from build123d import *

# Parameters (mm, degrees)
SKETCH1_W                = 250
SKETCH1_H                = 115
SKETCH1_R                = 8.5
SKETCH1_W_2              = 83
SKETCH1_H_2              = 55
BOSS_EXTRUDE1_DEPTH      = 10
SKETCH2_W                = 230
SKETCH2_H                = 95
SKETCH2_W_2              = 214
SKETCH2_H_2              = 79
BOSS_EXTRUDE2_DEPTH      = 15
SKETCH3_W                = 25
SKETCH3_H                = 25
CUT_EXTRUDE1_DEPTH       = 7
SKETCH4_W                = 93
SKETCH4_H                = 65
SKETCH4_W_2              = 83
SKETCH4_H_2              = 55
CUT_EXTRUDE2_DEPTH       = 5
SKETCH5_W                = 7
SKETCH5_H                = 5
SKETCH5_W_2              = 10
BOSS_EXTRUDE3_DEPTH      = 8
SKETCH7_W                = 7
SKETCH7_H                = 30
SKETCH7_W_2              = 10
BOSS_EXTRUDE4_DEPTH      = 5
SKETCH8_W                = 5.6
SKETCH8_H                = 2.8
CUT_EXTRUDE7_DEPTH       = 6.6
SKETCH9_W                = 5.6
SKETCH9_H                = 2.8
CUT_EXTRUDE8_DEPTH       = 6.6
CUT_EXTRUDE9_DEPTH       = 139.38457284
CUT_EXTRUDE9_DEPTH_BACK  = 139.38457284
SKETCH10_R               = 1.65
SKETCH11_R               = 1.65
BOSS_EXTRUDE5_DEPTH      = 3
SKETCH12_W               = 10
SKETCH12_H               = 0.5
CUT_EXTRUDE10_DEPTH      = 3
SKETCH13_W               = 30
SKETCH13_H               = 8
CUT_EXTRUDE11_DEPTH      = 6
SKETCH14_W               = 5.6
SKETCH14_H               = 2.8
CUT_EXTRUDE12_DEPTH      = 6.6
CUT_EXTRUDE13_DEPTH      = 139.222610307
CUT_EXTRUDE13_DEPTH_BACK = 139.222610307
SKETCH15_R               = 1.65
SKETCH16_W               = 5.6
SKETCH16_H               = 2.8
CUT_EXTRUDE14_DEPTH      = 6.6
CUT_EXTRUDE15_DEPTH      = 139.222610307
CUT_EXTRUDE15_DEPTH_BACK = 139.222610307
SKETCH17_R               = 1.65
SKETCH18_R               = 1.65
BOSS_EXTRUDE6_DEPTH      = 4
CHAMFER1_SIZE            = 15
CHAMFER2_SIZE            = 5
FILLET1_R                = 5


with BuildPart() as part:
    # Sketch1 → Boss-Extrude1 (new body)
    with BuildSketch(Plane(origin=(0, 0, 0), x_dir=(1, 0, 0), z_dir=(0, 1, 0))):
        Rectangle(SKETCH1_W, SKETCH1_H)
        with Locations(Location((23, 15, 0), (0, 0, 270))):
            Circle(SKETCH1_R, mode=Mode.SUBTRACT)
        with Locations(Location((58, 15, 0), (0, 0, 270))):
            Circle(SKETCH1_R, mode=Mode.SUBTRACT)
        with Locations(Location((23, -15, 0), (0, 0, 270))):
            Circle(SKETCH1_R, mode=Mode.SUBTRACT)
        with Locations(Location((58, -15, 0), (0, 0, 270))):
            Circle(SKETCH1_R, mode=Mode.SUBTRACT)
        with Locations(Location((93, 0, 0), (0, 0, 270))):
            Circle(SKETCH1_R, mode=Mode.SUBTRACT)
        with Locations((-53.5, 0)):
            Rectangle(SKETCH1_W_2, SKETCH1_H_2, mode=Mode.SUBTRACT)
    extrude(amount=BOSS_EXTRUDE1_DEPTH)

    # Sketch2 → Boss-Extrude2 (add)
    with BuildSketch(Plane.XZ):
        Rectangle(SKETCH2_W, SKETCH2_H)
        Rectangle(SKETCH2_W_2, SKETCH2_H_2, mode=Mode.SUBTRACT)
    extrude(amount=BOSS_EXTRUDE2_DEPTH)

    # Sketch3 → Cut-Extrude1 (cut)
    with BuildSketch(Plane.XZ):
        with Locations((23, 15)):
            Rectangle(SKETCH3_W, SKETCH3_H)
        with Locations((58, 15)):
            Rectangle(SKETCH3_W, SKETCH3_H)
        with Locations((23, -15)):
            Rectangle(SKETCH3_W, SKETCH3_H)
        with Locations((58, -15)):
            Rectangle(SKETCH3_W, SKETCH3_H)
        with Locations((93, 0)):
            Rectangle(SKETCH3_W, SKETCH3_H)
    extrude(amount=-CUT_EXTRUDE1_DEPTH, mode=Mode.SUBTRACT)

    # Sketch4 → Cut-Extrude2 (cut)
    with BuildSketch(Plane.XZ):
        with Locations((-53.5, 0)):
            Rectangle(SKETCH4_W, SKETCH4_H)
        with Locations((-53.5, 0)):
            Rectangle(SKETCH4_W_2, SKETCH4_H_2, mode=Mode.SUBTRACT)
    extrude(amount=-CUT_EXTRUDE2_DEPTH, mode=Mode.SUBTRACT)

    # Sketch5 → Boss-Extrude3 (add)
    with BuildSketch(Plane.XZ):
        with Locations((-103.5, 17.5)):
            Rectangle(SKETCH5_W, SKETCH5_H)
        with Locations((-103.5, -17.5)):
            Rectangle(SKETCH5_W, SKETCH5_H)
        with Locations((-2, 17.853765276)):
            Rectangle(SKETCH5_W_2, SKETCH5_H)
        with Locations((-2, -17.146234724)):
            Rectangle(SKETCH5_W_2, SKETCH5_H)
    extrude(amount=BOSS_EXTRUDE3_DEPTH)

    # Sketch7 → Boss-Extrude4 (add)
    with BuildSketch(Plane.XZ):
        with Locations((-103.5, 0)):
            Rectangle(SKETCH7_W, SKETCH7_H)
        with Locations((-2, 0.353765276)):
            Rectangle(SKETCH7_W_2, SKETCH7_H)
    extrude(amount=BOSS_EXTRUDE4_DEPTH)

    # Sketch8 → Cut-Extrude7 (cut)
    with BuildSketch(Plane.ZY.offset(7)):
        with Locations((0, -1.6)):
            Rectangle(SKETCH8_W, SKETCH8_H)
    extrude(amount=-CUT_EXTRUDE7_DEPTH, mode=Mode.SUBTRACT)

    # Sketch9 → Cut-Extrude8 (cut)
    with BuildSketch(Plane(origin=(-100, 0, 0), x_dir=(0, 0, -1), z_dir=(1, 0, 0))):
        with Locations((0, -1.6)):
            Rectangle(SKETCH9_W, SKETCH9_H)
    extrude(amount=-CUT_EXTRUDE8_DEPTH, mode=Mode.SUBTRACT)

    # Sketch10 → Cut-Extrude9 (cut, two sides: drawn at the far end of the back side and taken through both)
    with BuildSketch(Plane.XZ.offset(0.2).offset(-CUT_EXTRUDE9_DEPTH_BACK)):
        with Locations(Location((-3.7, 0, 0), (0, 0, 270))):
            Circle(SKETCH10_R)
        with Locations(Location((-103.478401375, 0, 0), (0, 0, 270))):
            Circle(SKETCH10_R)
    extrude(amount=CUT_EXTRUDE9_DEPTH + CUT_EXTRUDE9_DEPTH_BACK, mode=Mode.SUBTRACT)

    # Sketch11 → Boss-Extrude5 (add)
    with BuildSketch(Plane(origin=(0, 10, 0), x_dir=(1, 0, 0), z_dir=(0, 1, 0))):
        with Locations(Location((-3.7, 0, 0), (0, 0, 270))):
            Circle(SKETCH11_R)
        with Locations(Location((-103.478401375, 0, 0), (0, 0, 270))):
            Circle(SKETCH11_R)
    extrude(amount=-BOSS_EXTRUDE5_DEPTH)

    # Sketch12 → Cut-Extrude10 (cut)
    with BuildSketch(Plane.XZ.offset(8)):
        with Locations((-2, -14.896234724)):
            Rectangle(SKETCH12_W, SKETCH12_H)
    extrude(amount=-CUT_EXTRUDE10_DEPTH, mode=Mode.SUBTRACT)

    # Sketch13 → Cut-Extrude11 (cut)
    with BuildSketch(Plane.XZ.offset(15)):
        with Locations((-65, 43.5)):
            Rectangle(SKETCH13_W, SKETCH13_H)
        with Locations((65, 43.5)):
            Rectangle(SKETCH13_W, SKETCH13_H)
        with Locations((-65, -43.5)):
            Rectangle(SKETCH13_W, SKETCH13_H)
        with Locations((65, -43.5)):
            Rectangle(SKETCH13_W, SKETCH13_H)
    extrude(amount=-CUT_EXTRUDE11_DEPTH, mode=Mode.SUBTRACT)

    # Sketch14 → Cut-Extrude12 (cut)
    with BuildSketch(Plane.XY.offset(47.5)):
        with Locations((-65, -4.6)):
            Rectangle(SKETCH14_W, SKETCH14_H)
        with Locations((65, -4.6)):
            Rectangle(SKETCH14_W, SKETCH14_H)
    extrude(amount=-CUT_EXTRUDE12_DEPTH, mode=Mode.SUBTRACT)

    # Sketch15 → Cut-Extrude13 (cut, two sides: drawn at the far end of the back side and taken through both)
    with BuildSketch(Plane.XZ.offset(3.2).offset(-CUT_EXTRUDE13_DEPTH_BACK)):
        with Locations(Location((-65, 44.2, 0), (0, 0, 270))):
            Circle(SKETCH15_R)
        with Locations(Location((65, 44.2, 0), (0, 0, 270))):
            Circle(SKETCH15_R)
    extrude(amount=CUT_EXTRUDE13_DEPTH + CUT_EXTRUDE13_DEPTH_BACK, mode=Mode.SUBTRACT)

    # Sketch16 → Cut-Extrude14 (cut)
    with BuildSketch(Plane(origin=(0, 0, -47.5), x_dir=(-1, 0, 0), z_dir=(0, 0, -1))):
        with Locations((-65, -4.6)):
            Rectangle(SKETCH16_W, SKETCH16_H)
        with Locations((65, -4.6)):
            Rectangle(SKETCH16_W, SKETCH16_H)
    extrude(amount=-CUT_EXTRUDE14_DEPTH, mode=Mode.SUBTRACT)

    # Sketch17 → Cut-Extrude15 (cut, two sides: drawn at the far end of the back side and taken through both)
    with BuildSketch(Plane.XZ.offset(3.2).offset(-CUT_EXTRUDE15_DEPTH_BACK)):
        with Locations(Location((65, -44.2, 0), (0, 0, 270))):
            Circle(SKETCH17_R)
        with Locations(Location((-65, -43.998374959, 0), (0, 0, 270))):
            Circle(SKETCH17_R)
    extrude(amount=CUT_EXTRUDE15_DEPTH + CUT_EXTRUDE15_DEPTH_BACK, mode=Mode.SUBTRACT)

    # Sketch18 → Boss-Extrude6 (add)
    with BuildSketch(Plane(origin=(0, 10, 0), x_dir=(1, 0, 0), z_dir=(0, 1, 0))):
        with Locations(Location((-65, 43.998374959, 0), (0, 0, 270))):
            Circle(SKETCH18_R)
        with Locations(Location((65, 44.2, 0), (0, 0, 270))):
            Circle(SKETCH18_R)
        with Locations(Location((-65, -44.2, 0), (0, 0, 270))):
            Circle(SKETCH18_R)
        with Locations(Location((65, -44.2, 0), (0, 0, 270))):
            Circle(SKETCH18_R)
    extrude(amount=-BOSS_EXTRUDE6_DEPTH)

    # Chamfer1
    chamfer1_edges = [part.edges().sort_by_distance(p)[0] for p in [
        (125, 5, 57.5),
        (-125, 5, 57.5),
        (-125, 5, -57.5),
        (125, 5, -57.5),
    ]]
    chamfer(chamfer1_edges, length=CHAMFER1_SIZE)

    # Chamfer2
    chamfer2_edges = [part.edges().sort_by_distance(p)[0] for p in [
        (-125, 10, 0),
        (0, 10, -57.5),
        (125, 10, 0),
        (0, 10, 57.5),
        (-117.5, 10, 50),
        (117.5, 10, 50),
        (117.5, 10, -50),
        (-117.5, 10, -50),
    ]]
    chamfer(chamfer2_edges, length=CHAMFER2_SIZE)

    # Fillet1
    fillet1_edges = [part.edges().sort_by_distance(p)[0] for p in [
        (115, -7.5, -47.5),
        (115, -7.5, 47.5),
        (-115, -7.5, 47.5),
        (-115, -7.5, -47.5),
    ]]
    fillet(fillet1_edges, radius=FILLET1_R)


solid = part.part
The listing builds one solid part. Answer for the finished solid, in the listing's coordinates (mm). A direction names the side the tool comes from. Coordinates: 2 decimals unless noted, no trailing zeros. Order: outer loops, then holes, each group sorted by start corner. A loop starts at its lowest first (then second) coordinate and runs counter-clockwise, first axis right, second up. Notation, with made-up numbers: M -34,84 L -24,84 A18 cw -24,104 Z; hole C -19.75,-5.5 d4. An arc over 180 degrees is marked long. Use CSV: the item, a comma, the result in double quotes.
Q1. Section B-B (x = -37) is taken. Determine the outline of the cut face in (y, z).
Here are the results:
outline,"M -15,-47.5 L 0,-47.5 L 0,-57.5 L 5,-57.5 L 10,-52.5 L 10,-27.5 L 5,-27.5 L 5,-32.5 L 0,-32.5 L 0,-39.5 L -15,-39.5 Z; M -15,39.5 L 0,39.5 L 0,32.5 L 5,32.5 L 5,27.5 L 10,27.5 L 10,52.5 L 5,57.5 L 0,57.5 L 0,47.5 L -15,47.5 Z"
Q2. Straight lines are drawn through the part: L1, parallel to X at y = -11.25, z = -43; L2, parallel to Z at x = -65, y = 0.5; L3, parallel to Z at x = 65, y = -1. For each, find the intervals that lie inside material, in ascending order.
Here are the results:
L1,"-114.97 to -80, -50 to 50, 80 to 114.97"
L2,"-57.5 to -45.65, -42.35 to -32.5, 32.5 to 42.55, 45.85 to 57.5"
L3,"-47.5 to -45.85, -42.55 to -39.5, 39.5 to 42.55, 45.85 to 47.5"
Q3. Section C-C (z = -35.5) is taken. Determine the outline of the cut face in (x, y).
Here are the results:
outline,"M -125,0 L -115,0 L -115,-15 L -107,-15 L -107,0 L 107,0 L 107,-15 L 115,-15 L 115,0 L 125,0 L 125,5 L 120,10 L -120,10 L -125,5 Z"
Q4. Section A-A (x = 23) is taken. Give the number of separate pieces and of enclosed holes in the cut face, then the cut area to 3 significant figures.
Here are the results:
separate pieces,"3"
enclosed holes,"0"
area,"913 mm2"
Q5. A tool of negligible diameter and unlimited length cuts with its end or side. For faces 1 (the flat face through (-80, -12, -44)), 2 (the flat face through (105.5, 3, 0)), 3 (the flat face through (-4, -3, -2)), from which of +Z, -Z, +X, -X, +Y, -Y can it reach the whole face along a straight path? Write none if from no direction.
Here are the results:
face 1,"+Z, -Z, -Y"
face 2,"-Y"
face 3,"none"
Q6. Determine the mould class of faces 4 (the flat face through (117.4, 2.5, 50.1)), 5 (the cylindrical face through (-113.57, -7.6, -46)), 6 (the flat face through (80, -12, -44)) for opening direction X: pulls with the +X half, pulls with the -X half, needs draft (parallel to the pull), parting line crosses it, or undercut.
Here are the results:
face 4,"pulls with the +X half"
face 5,"pulls with the -X half"
face 6,"undercut"
Q7. Given pin 1 Ø7.5 at (x, z) = (26, 10) entering from -Y; pin 2 Ø6 at (x, y) = (32.5, -8) entering from +Z; pin 3 Ø4 at (x, y) = (-59, 8) entering from -Z, each flat-ended and moving along its own axis, determine where each tip first touches the part or whether it passes through.
Here are the results:
pin 1,"y = 7"
pin 2,"z = 47.5"
pin 3,"z = -56.5"
